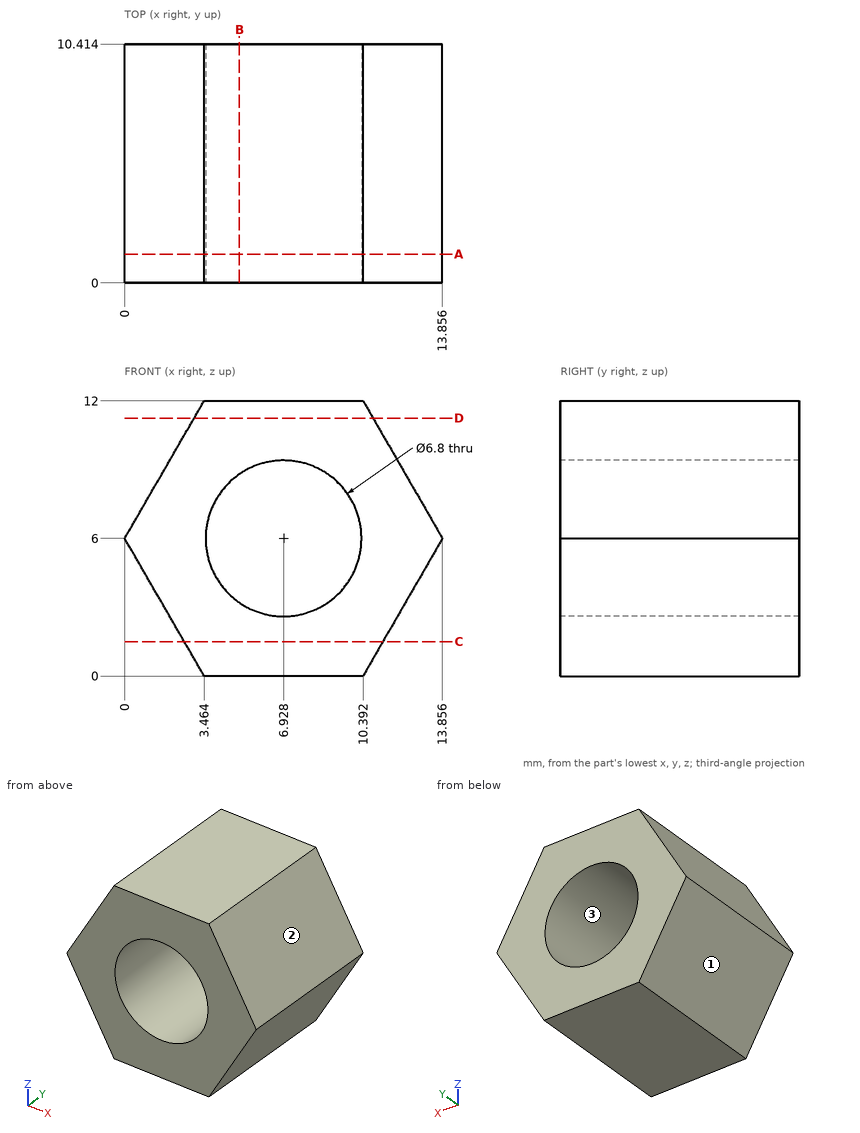
Geometry check sheet. Reference: drawing and pictorial views, mm from the part's lowest x, y, z. Give positions to 0.01 mm unless a question says otherwise; leave off trailing zeros. Write each loop counter-clockwise with the first axis right and the second up, starting at its lowest first coordinate (ties: lowest second). Pieces come first, ordered by that corner, then holes. Notation, with made-up numbers: M 84,72 L 130,72 A21 ccw 130,96 Z; hole C -26.75,-5.5 d11. An arc over 180 degrees is marked long. Answer as CSV lines item,"result". Start each with the question number.
Q1. Section check A-A, the plane y = 1.25. Record the cut outline in (x, z).
Q2. Section check B-B, the plane x = 5. Record the cut outline in (y, z).
Q3. Section check D-D, the plane z = 11.25. Record the cut outline in (x, y) (1 decimal).
Q4. Material ranges on L1, parallel to Z at x = 4.5, y = 7.75; L2, parallel to Z at x = 5.5, y = 5.5 (1 decimal); L3, parallel to X at y = 8.5, z = 9 (1 decimal), recorded low to high.
Q5. Section check C-C, the plane z = 1.5. Record the cut outline in (x, y), then the cut area to 3 significant figures.
Q6. Release check for a two-part mould opening along Z. For the marked faces 1, 2 and 3 record: pulls with the +Z half, pulls with the -Z half, needs draft (parallel to the pull), parting line crosses it, or undercut.
Geometry says:
1,outline,"M 0,6 L 3.46,0 L 10.39,0 L 13.86,6 L 10.39,12 L 3.46,12 Z; hole C 6.93,6 d6.8"
2,outline,"M 0,0 L 10.41,0 L 10.41,3.2 L 0,3.2 Z; M 0,8.8 L 10.41,8.8 L 10.41,12 L 0,12 Z"
3,outline,"M 3,0 L 10.8,0 L 10.8,10.4 L 3,10.4 Z"
4,L1,"0 to 3.62, 8.38 to 12"
4,L2,"0 to 2.9, 9.1 to 12"
4,L3,"1.7 to 5.3, 8.5 to 12.1"
5,outline,"M 2.6,0 L 11.26,0 L 11.26,10.41 L 2.6,10.41 Z"
5,area,"90.2 mm^2"
6,face 1,"pulls with the -Z half"
6,face 2,"pulls with the +Z half"
6,face 3,"undercut"
